Answer from the drawing. Dimensions are ordinates in mm from the lowest x, y and z of the part. A direction names the side the tool comes from. Coordinates: 2 decimals unless noted, no trailing zeros. Order: outer loops, then holes, each group sorted by start corner. A loop starts at its lowest first (then second) coordinate and runs counter-clockwise, first axis right, second up. Notation, with made-up numbers: (29, 76) - (57, 76) arc R29 ccw to (57, 112) - close; hole circle Ø8 at (55, 32). An arc over 180 degrees is marked (long way). Use a Markdown table: item, result. Add a question column.
Item 1: Flat-ended cylindrical pins translate along their axes: P1, Ø22, axis at y = 8.5, z = 30.5, coming from the +X side; P2, Ø8, axis at y = 25, z = 46.5, coming from the +X side; P3, Ø13.5, axis at x = 58, z = 44.5, coming from the -Y side. Find the tip coordinate at first contact, or state that the pin passes through.
Item 2: Find the intervals of material crossed by line 1 along Z through (x, y) = (84, 28.5); line 2 along Y through (x, z) = (77.5, 85.5); line 3 along Z through (x, y) = (21.5, 14.5), in increasing order.
Item 3: The part is cut by section D-D, the plane y = 40. Give the vertices of the cut face in (x, z).
Item 4: The part is cut by section C-C, the plane z = 25.5. Give the vertices of the cut face in (x, y), then the cut area to 3 significant figures.
Item 5: The part is cut by section B-B, the plane x = 70.5. Give the vertices of the cut face in (y, z).
Item 6: The part is cut by section A-A, the plane z = 73. Give the vertices of the cut face in (x, y), then the cut area to 3 significant figures.
Item 7: For the marked faces 1, 2, 3, 4 and 5, determine the directions among +Z, -Z, +X, -X, +Y, -Y from which every point of the face is accessible in a straight line to the end or side of a thin tool.
Item 8: The mould has two halves that part along X. Classify the marked faces 6, 7 and 8: released by +X, released by -X, zero draft, split by the parting line, or undercut.
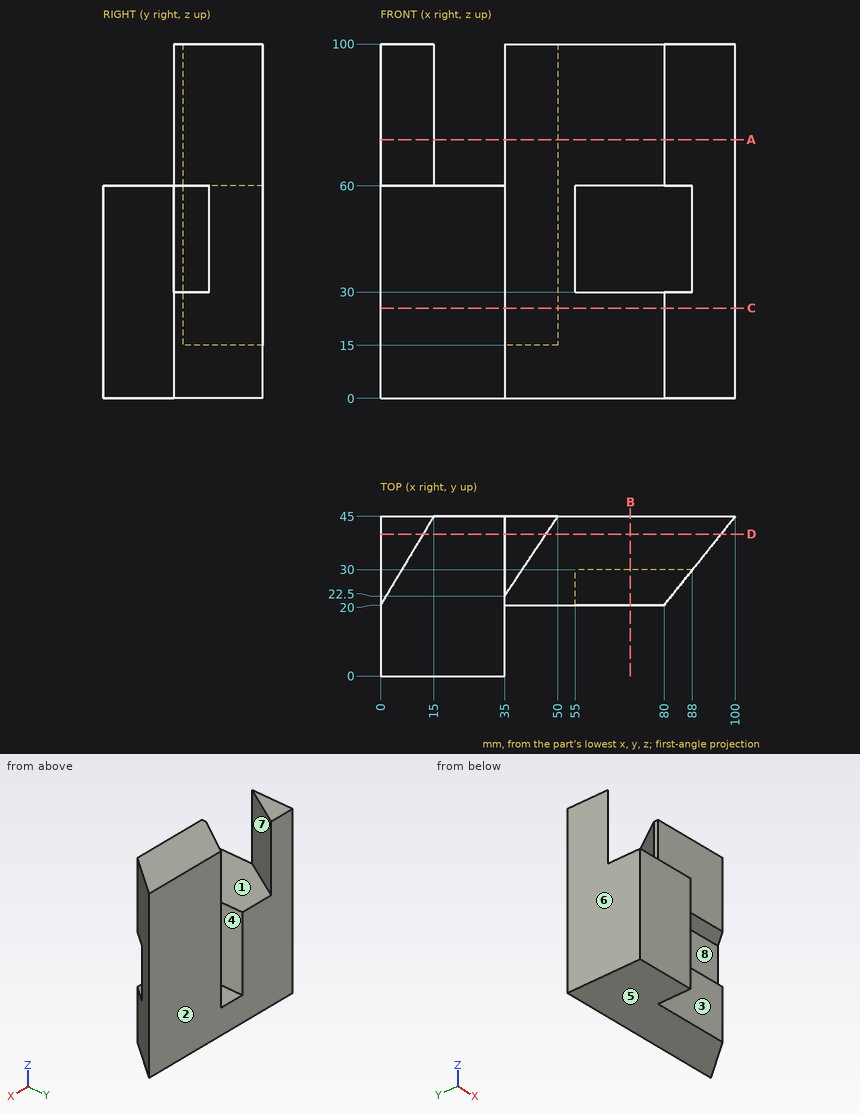
Solution:
| question | item | result |
|---|---|---|
| 1 | P1 | stops at x = 35 |
| 1 | P2 | stops at x = 55 |
| 1 | P3 | stops at y = 20 |
| 2 | line 1 | z = 0 to 30, 60 to 100 |
| 2 | line 2 | y = 20 to 45 |
| 2 | line 3 | z = 0 to 60 |
| 3 | outline | (0, 0) - (96, 0) - (96, 100) - (46.67, 100) - (46.67, 15) - (35, 15) - (35, 60) - (12, 60) - (12, 100) - (0, 100) - close |
| 4 | outline | (0, 0) - (35, 0) - (35, 20) - (80, 20) - (100, 45) - (50, 45) - (35, 22.5) - (35, 45) - (0, 45) - close |
| 4 | area | 2,780 mm2 |
| 5 | outline | (20, 0) - (45, 0) - (45, 100) - (20, 100) - (20, 60) - (30, 60) - (30, 30) - (20, 30) - close |
| 6 | outline | (0, 20) - (15, 45) - (0, 45) - close; (35, 20) - (80, 20) - (100, 45) - (50, 45) - (35, 22.5) - close |
| 6 | area | 1,390 mm2 |
| 7 | face 1 | +Z, -Y |
| 7 | face 2 | +Z, -Z, +X, -X, +Y |
| 7 | face 3 | +Z, -Z, +X, -Y |
| 7 | face 4 | +Z, +Y |
| 7 | face 5 | -Z, +X, -X, +Y, -Y |
| 8 | face 6 | released by -X |
| 8 | face 7 | undercut |
| 8 | face 8 | zero draft |
